Input: part model. Units: mm. Frame: model coordinates. Face numbers are marked on the shaded views. Round coordinates to 2 decimals unless told otherwise and drop trailing zeros. Loops run counter-clockwise (first coordinate to the right, second up) from the corner with the lowest first, then second, coordinate; pieces in that order, holes last. Notation, with made-up numbers: (-9.75, 22.25) -> (12.25, 22.25) arc R35 ccw to (12.25, 59.25) -> close; hole circle Ø7 at (21, 13.5). An arc over 180 degrees is marked (long way). Answer as a JSON object with one key per item and string values. Group by question number.
Item 1: Section query B-B on x = 0. Return loops of the section in (y, z), and give its area (3 significant figures).
Item 2: Pin query (flat end, axial travel): pin 1 (1 mm diameter, centred on y = 1.5, z = 17, fed in from +X); pin 2 (1.5 mm diameter, centred on x = -20.5, y = 0.5, fed in from -Z); pin 3 (1.5 mm diameter, centred on x = 20.5, y = 2, fed in from +Z); pin 4 (2.5 mm diameter, centred on x = 0, z = 25, fed in from -Y). Return the tip coordinate at first contact, or that it passes through.
Item 3: Material intervals for line 1 (X direction, y = 1, z = 0); line 2 (X direction, y = 2.85, z = 25); line 3 (Z direction, x = -12, y = 3.55), sorted ascending. Write a range as [from, to].
Item 4: Section query A-A on z = 0. Return loops of the section in (x, y).
Item 5: Draft query along X for the marked faces 1 and 2. Return one class per face: released by +X, released by -X, zero draft, split by the parting line, or undercut.
Item 6: Section query C-C on y = 3.1. Return loops of the section in (x, z).
from build123d import *

# Parameters (mm, degrees)
CSK_SLOT_FOR_M4_COUNTERSUNK_FLAT_HEA_2_COUNT = 2
CSK_SLOT_FOR_M4_COUNTERSUNK_FLAT_HEA_2_PITCH = 50
FILLET1_R                                    = 1
CUT_EXTRUDE2_START                           = -10
SKETCH5_R                                    = 17
CUT_EXTRUDE2_DEPTH                           = 10


with BuildPart() as part:
    # Sketch1 → Revolve1 (revolve)
    with BuildSketch(Plane.XY, mode=Mode.PRIVATE) as revolve1_sk:
        Polygon((-32.5, 0), (-32.5, 4), (-17, 4), (-17, 2), (0, 2), (0, 0), align=None)
    revolve(revolve1_sk.sketch.rotate(Axis((0, 0, 0), (0, -1, 0)), 270), axis=Axis((0, 0, 0), (0, -1, 0)))

    # Sketch3 → CSK SLOT for M4 Countersunk Flat Head Screw1 (revolve, cut)
    with BuildSketch(Plane(origin=(0, 0, 25), x_dir=(0, 0, -1), z_dir=(1, 0, 0))):
        Polygon((0, 0), (0, 4), (2.25, 4), (2.25, 2.45), (4.7, 0), align=None)
    csk_slot_for_m4_countersunk_flat_head_sc = revolve(axis=Axis((0, -6.35, 25), (0, 1, 0)), mode=Mode.SUBTRACT)

    # CSK SLOT for M4 Countersunk Flat Hea 2: CSK SLOT for M4 Countersunk Flat Head Screw1 ×2
    with Locations(*[(0, 0, -i * CSK_SLOT_FOR_M4_COUNTERSUNK_FLAT_HEA_2_PITCH) for i in range(1, CSK_SLOT_FOR_M4_COUNTERSUNK_FLAT_HEA_2_COUNT)]):
        add(csk_slot_for_m4_countersunk_flat_head_sc, mode=Mode.SUBTRACT)

    # Fillet1
    fillet1_edges = [part.edges().sort_by_distance(p)[0] for p in [
        (0, 2, -17),
        (0, 0, -32.5),
    ]]
    fillet(fillet1_edges, radius=FILLET1_R)

    # Sketch5 → Cut-Extrude2 (cut)
    with BuildSketch(Plane(origin=(0, 4, 0), x_dir=(1, 0, 0), z_dir=(0, 1, 0)).offset(CUT_EXTRUDE2_START)):
        with Locations(Location((0, 0, 0), (0, 0, 270))):
            Circle(SKETCH5_R)
    extrude(amount=CUT_EXTRUDE2_DEPTH, mode=Mode.SUBTRACT)


solid = part.part
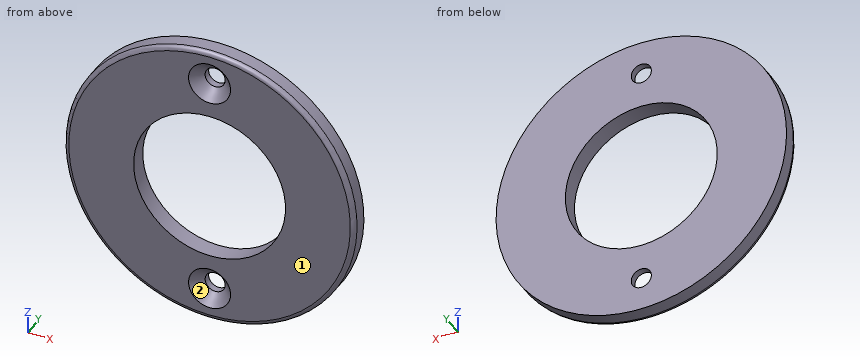
Solved:
{
 "1": {"outline": "(0, -31.5) arc R1 ccw to (1, -32.5) -> (4, -32.5) -> (4, -27.25) -> (2.45, -27.25) -> (0, -29.7) -> close; (0, -20.3) -> (2.45, -22.75) -> (4, -22.75) -> (4, -17) -> (0, -17) -> close; (0, 17) -> (4, 17) -> (4, 22.75) -> (2.45, 22.75) -> (0, 20.3) -> close; (0, 29.7) -> (2.45, 27.25) -> (4, 27.25) -> (4, 32.5) -> (1, 32.5) arc R1 ccw to (0, 31.5) -> close", "area": "75.6 mm²"},
 "2": {"pin 1": "x = 28", "pin 2": "z = -25.74", "pin 3": "z = 25.81", "pin 4": "through"},
 "3": {"line 1": "[-32.5, -17], [17, 32.5]", "line 2": "[-20.77, -2.25], [2.25, 20.77]", "line 3": "[-30.2, -12.04], [12.04, 30.2]"},
 "4": {"outline": "(-32.5, 1) arc R1 ccw to (-31.5, 0) -> (-17, 0) -> (-17, 4) -> (-32.5, 4) -> close; (17, 0) -> (31.5, 0) arc R1 ccw to (32.5, 1) -> (32.5, 4) -> (17, 4) -> close"},
 "5": {"face 1": "zero draft", "face 2": "undercut"},
 "6": {"outline": "circle Ø65 at (0, 0); hole circle Ø34 at (0, 0); hole circle Ø4.5 at (0, -25); hole circle Ø4.5 at (0, 25)"}
}
